CAD build for the part. Positions are in the model's coordinates, mm. A direction names the side the tool comes from. Give positions to 0.01 mm unless a question says otherwise; leave off trailing zeros. Write each loop counter-clockwise with the first axis right and the second up, starting at its lowest first coordinate (ties: lowest second). Pieces come first, ordered by that corner, then holes. Notation, with made-up numbers: (30.5, 44) - (71.5, 44) arc R24 cw to (71.5, 63) - close; hole circle Ø6 at (-31.5, 47). An arc over 180 degrees is marked (long way). Put each result on its own line as item: value. Start each with the question number.
1. Tool access for faces 5 (the flat face through (0, -5, 6)), 6 (the flat face through (0, -5, -6)), 7 (the flat face through (18, -5, -4)): list every direction of +Z, -Z, +X, -X, +Y, -Y with a clear straight run to the whole face (end or side of a thin tool).
2. Cut at C-C on y = -5. List the corners of the cut face in (x, z).
3. Cut at D-D on z = 3.5. List the corners of the cut face in (x, y), and give its area (3 significant figures).
4. Drop flat-ended pins along their axis: pin 1 (3 mm diameter, centred on x = -18, y = -5, fed in from +Z); pin 2 (3 mm diameter, centred on x = 18.5, y = -3.5, fed in from +Z); pin 3 (3 mm diameter, centred on x = 1, y = -7, fed in from -Z). Give the stop position or say it passes through.
5. Mould opens along Y. For faces 1 (the cylindrical face through (-15.715, -4.28, 1.07)), 2 (the flat face through (-18, -5, -4)), 3 (the flat face through (-19, -5, -22)), 4 (the flat face through (0, 0, -5)) say: +Y half, -Y half, draft (parallel to the pull), parting line (faces both ways), or undercut.
6. Cut at A-A on x = -18. List the corners of the cut face in (y, z).
7. Cut at B-B on z = -6.5. List the corners of the cut face in (x, y).
8. Wall check: line 1 (X direction, y = -2.5, z = -17); line 2 (Y direction, x = -18, z = 2.75); line 3 (Y direction, x = 18, z = 3.75). Give the ranges that are in metal, low to high.
from build123d import *

# Parameters (mm, degrees)
F0_W     = 8
F0_H     = 16
F1_DEPTH = 10
F2_R     = 2.395941
F2_R_2   = 2.897802
F3_DEPTH = 10


with BuildPart() as f1:
    # F0 (on Front) → F1 (new body)
    with BuildSketch(Plane.XZ):
        Polygon((23, 6), (-23, 6), (-23, -6), (-15, -6), (15, -6), (23, -6), align=None)
        with Locations((-19, -14)):
            Rectangle(F0_W, F0_H)
        with Locations((19, -14)):
            Rectangle(F0_W, F0_H)
    extrude(amount=F1_DEPTH)

    # F2 (on face) → F3 (cut)
    with BuildSketch(Plane.XY.offset(6)):
        with Locations((-18, -5)):
            Circle(F2_R)
        with Locations((18, -5)):
            Circle(F2_R_2)
    extrude(amount=-F3_DEPTH, mode=Mode.SUBTRACT)


solid = f1.part
Report:
1. face 5: +Z, +X, -X, +Y, -Y
1. face 6: -Z, +Y, -Y
1. face 7: +Z
2. outline: (-23, -22) - (-15, -22) - (-15, -6) - (15, -6) - (15, -22) - (23, -22) - (23, 6) - (20.9, 6) - (20.9, -4) - (15.1, -4) - (15.1, 6) - (-15.6, 6) - (-15.6, -4) - (-20.4, -4) - (-20.4, 6) - (-23, 6) - close
3. outline: (-23, -10) - (23, -10) - (23, 0) - (-23, 0) - close; hole circle Ø4.79 at (-18, -5); hole circle Ø5.8 at (18, -5)
3. area: 416 mm²
4. pin 1: stops at z = -4
4. pin 2: stops at z = 6
4. pin 3: stops at z = -6
5. face 1: undercut
5. face 2: undercut
5. face 3: draft
5. face 4: +Y half
6. outline: (-10, -22) - (0, -22) - (0, 6) - (-2.6, 6) - (-2.6, -4) - (-7.4, -4) - (-7.4, 6) - (-10, 6) - close
7. outline: (-23, -10) - (-15, -10) - (-15, 0) - (-23, 0) - close; (15, -10) - (23, -10) - (23, 0) - (15, 0) - close
8. line 1: x = -23 to -15, 15 to 23
8. line 2: y = -10 to -7.4, -2.6 to 0
8. line 3: y = -10 to -7.9, -2.1 to 0
